For this review, take the finished solid that the model builds, in its own axes (mm). Face numbers are marked on the shaded views. Coordinates: 2 decimals unless noted, no trailing zeros. Loops run counter-clockwise (first coordinate to the right, second up) from the corner with the lowest first, then second, coordinate; pieces in that order, holes last.
```python
from build123d import *

# Parameters (mm, degrees)
SKETCH1_W           = 277
SKETCH1_H           = 3
BOSS_EXTRUDE1_DEPTH = 450
CUT_EXTRUDE1_REACH  = 520.295
SKETCH2_W           = 6
SKETCH2_H           = 250
CUT_EXTRUDE2_REACH  = 520.295
SKETCH3_R           = 1.55
SKETCH4_W           = 7
SKETCH4_H           = 75
SKETCH4_W_2         = 5
SKETCH4_H_2         = 35
BOSS_EXTRUDE2_DEPTH = 3


with BuildPart() as part:
    # Sketch1 → Boss-Extrude1 (new body)
    with BuildSketch(Plane.XY):
        with Locations((-118.640040599, -13.427850278)):
            Rectangle(SKETCH1_W, SKETCH1_H)
    extrude(amount=BOSS_EXTRUDE1_DEPTH)

    # Sketch2 → Cut-Extrude1 (cut, up to next)
    with BuildSketch(Plane(origin=(0, -11.927850278, 0), x_dir=(1, 0, 0), z_dir=(0, 1, 0)), mode=Mode.PRIVATE) as cut_extrude1_sk1:
        with Locations((-234.140040599, -225)):
            Rectangle(SKETCH2_W, SKETCH2_H)
    cut_extrude1_tool1 = extrude(cut_extrude1_sk1.sketch, amount=-CUT_EXTRUDE1_REACH, mode=Mode.PRIVATE) & part.part
    # Sketch2 → Cut-Extrude1 (cut, up to next)
    with BuildSketch(Plane(origin=(0, -11.927850278, 0), x_dir=(1, 0, 0), z_dir=(0, 1, 0)), mode=Mode.PRIVATE) as cut_extrude1_sk2:
        with Locations((-3.140040599, -225)):
            Rectangle(SKETCH2_W, SKETCH2_H)
    cut_extrude1_tool2 = extrude(cut_extrude1_sk2.sketch, amount=-CUT_EXTRUDE1_REACH, mode=Mode.PRIVATE) & part.part
    add(cut_extrude1_tool1.solids().sort_by_distance((-234.140041, -11.92785, 225))[0], mode=Mode.SUBTRACT)
    add(cut_extrude1_tool2.solids().sort_by_distance((-3.140041, -11.92785, 225))[0], mode=Mode.SUBTRACT)

    # Sketch3 → Cut-Extrude2 (cut, up to next)
    with BuildSketch(Plane(origin=(0, -11.927850278, 0), x_dir=(1, 0, 0), z_dir=(0, 1, 0)), mode=Mode.PRIVATE) as cut_extrude2_sk1:
        with Locations(Location((-102.460040599, -431.322984009, 0), (0, 0, 180))):
            Circle(SKETCH3_R)
    cut_extrude2_tool1 = extrude(cut_extrude2_sk1.sketch, amount=-CUT_EXTRUDE2_REACH, mode=Mode.PRIVATE) & part.part
    # Sketch3 → Cut-Extrude2 (cut, up to next)
    with BuildSketch(Plane(origin=(0, -11.927850278, 0), x_dir=(1, 0, 0), z_dir=(0, 1, 0)), mode=Mode.PRIVATE) as cut_extrude2_sk2:
        with Locations(Location((-75.460040599, -442.983238046, 0), (0, 0, 180))):
            Circle(SKETCH3_R)
    cut_extrude2_tool2 = extrude(cut_extrude2_sk2.sketch, amount=-CUT_EXTRUDE2_REACH, mode=Mode.PRIVATE) & part.part
    # Sketch3 → Cut-Extrude2 (cut, up to next)
    with BuildSketch(Plane(origin=(0, -11.927850278, 0), x_dir=(1, 0, 0), z_dir=(0, 1, 0)), mode=Mode.PRIVATE) as cut_extrude2_sk3:
        with Locations(Location((-92.910040599, -383.404829271, 0), (0, 0, 180))):
            Circle(SKETCH3_R)
    cut_extrude2_tool3 = extrude(cut_extrude2_sk3.sketch, amount=-CUT_EXTRUDE2_REACH, mode=Mode.PRIVATE) & part.part
    # Sketch3 → Cut-Extrude2 (cut, up to next)
    with BuildSketch(Plane(origin=(0, -11.927850278, 0), x_dir=(1, 0, 0), z_dir=(0, 1, 0)), mode=Mode.PRIVATE) as cut_extrude2_sk4:
        with Locations(Location((10.539959401, -350.404829271, 0), (0, 0, 180))):
            Circle(SKETCH3_R)
    cut_extrude2_tool4 = extrude(cut_extrude2_sk4.sketch, amount=-CUT_EXTRUDE2_REACH, mode=Mode.PRIVATE) & part.part
    # Sketch3 → Cut-Extrude2 (cut, up to next)
    with BuildSketch(Plane(origin=(0, -11.927850278, 0), x_dir=(1, 0, 0), z_dir=(0, 1, 0)), mode=Mode.PRIVATE) as cut_extrude2_sk5:
        with Locations(Location((-7.460040599, -444.433238046, 0), (0, 0, 180))):
            Circle(SKETCH3_R)
    cut_extrude2_tool5 = extrude(cut_extrude2_sk5.sketch, amount=-CUT_EXTRUDE2_REACH, mode=Mode.PRIVATE) & part.part
    # Sketch3 → Cut-Extrude2 (cut, up to next)
    with BuildSketch(Plane(origin=(0, -11.927850278, 0), x_dir=(1, 0, 0), z_dir=(0, 1, 0)), mode=Mode.PRIVATE) as cut_extrude2_sk6:
        with Locations(Location((-247.340040599, -350.40562763, 0), (0, 0, 180))):
            Circle(SKETCH3_R)
    cut_extrude2_tool6 = extrude(cut_extrude2_sk6.sketch, amount=-CUT_EXTRUDE2_REACH, mode=Mode.PRIVATE) & part.part
    # Sketch3 → Cut-Extrude2 (cut, up to next)
    with BuildSketch(Plane(origin=(0, -11.927850278, 0), x_dir=(1, 0, 0), z_dir=(0, 1, 0)), mode=Mode.PRIVATE) as cut_extrude2_sk7:
        with Locations(Location((-229.340040599, -444.434036405, 0), (0, 0, 180))):
            Circle(SKETCH3_R)
    cut_extrude2_tool7 = extrude(cut_extrude2_sk7.sketch, amount=-CUT_EXTRUDE2_REACH, mode=Mode.PRIVATE) & part.part
    # Sketch3 → Cut-Extrude2 (cut, up to next)
    with BuildSketch(Plane(origin=(0, -11.927850278, 0), x_dir=(1, 0, 0), z_dir=(0, 1, 0)), mode=Mode.PRIVATE) as cut_extrude2_sk8:
        with Locations(Location((-161.340040599, -442.984036405, 0), (0, 0, 180))):
            Circle(SKETCH3_R)
    cut_extrude2_tool8 = extrude(cut_extrude2_sk8.sketch, amount=-CUT_EXTRUDE2_REACH, mode=Mode.PRIVATE) & part.part
    # Sketch3 → Cut-Extrude2 (cut, up to next)
    with BuildSketch(Plane(origin=(0, -11.927850278, 0), x_dir=(1, 0, 0), z_dir=(0, 1, 0)), mode=Mode.PRIVATE) as cut_extrude2_sk9:
        with Locations(Location((-134.340040599, -431.323782367, 0), (0, 0, 180))):
            Circle(SKETCH3_R)
    cut_extrude2_tool9 = extrude(cut_extrude2_sk9.sketch, amount=-CUT_EXTRUDE2_REACH, mode=Mode.PRIVATE) & part.part
    # Sketch3 → Cut-Extrude2 (cut, up to next)
    with BuildSketch(Plane(origin=(0, -11.927850278, 0), x_dir=(1, 0, 0), z_dir=(0, 1, 0)), mode=Mode.PRIVATE) as cut_extrude2_sk10:
        with Locations(Location((-143.890040599, -383.40562763, 0), (0, 0, 180))):
            Circle(SKETCH3_R)
    cut_extrude2_tool10 = extrude(cut_extrude2_sk10.sketch, amount=-CUT_EXTRUDE2_REACH, mode=Mode.PRIVATE) & part.part
    add(cut_extrude2_tool1.solids().sort_by_distance((-102.460041, -11.92785, 431.322984))[0], mode=Mode.SUBTRACT)
    add(cut_extrude2_tool2.solids().sort_by_distance((-75.460041, -11.92785, 442.983238))[0], mode=Mode.SUBTRACT)
    add(cut_extrude2_tool3.solids().sort_by_distance((-92.910041, -11.92785, 383.404829))[0], mode=Mode.SUBTRACT)
    add(cut_extrude2_tool4.solids().sort_by_distance((10.539959, -11.92785, 350.404829))[0], mode=Mode.SUBTRACT)
    add(cut_extrude2_tool5.solids().sort_by_distance((-7.460041, -11.92785, 444.433238))[0], mode=Mode.SUBTRACT)
    add(cut_extrude2_tool6.solids().sort_by_distance((-247.340041, -11.92785, 350.405628))[0], mode=Mode.SUBTRACT)
    add(cut_extrude2_tool7.solids().sort_by_distance((-229.340041, -11.92785, 444.434036))[0], mode=Mode.SUBTRACT)
    add(cut_extrude2_tool8.solids().sort_by_distance((-161.340041, -11.92785, 442.984036))[0], mode=Mode.SUBTRACT)
    add(cut_extrude2_tool9.solids().sort_by_distance((-134.340041, -11.92785, 431.323782))[0], mode=Mode.SUBTRACT)
    add(cut_extrude2_tool10.solids().sort_by_distance((-143.890041, -11.92785, 383.405628))[0], mode=Mode.SUBTRACT)

    # Sketch4 → Boss-Extrude2 (add)
    with BuildSketch(Plane.XZ.offset(14.927850278)):
        with Locations((-253.640040599, 412.5)):
            Rectangle(SKETCH4_W, SKETCH4_H)
        with Locations((16.359959401, 412.5)):
            Rectangle(SKETCH4_W, SKETCH4_H)
        with Locations((-253.640040599, 37.5)):
            Rectangle(SKETCH4_W, SKETCH4_H)
        with Locations((16.359959401, 37.5)):
            Rectangle(SKETCH4_W, SKETCH4_H)
        with Locations((-118.640040599, 217.477852068)):
            Rectangle(SKETCH4_W_2, SKETCH4_H_2)
    extrude(amount=BOSS_EXTRUDE2_DEPTH)


solid = part.part
```
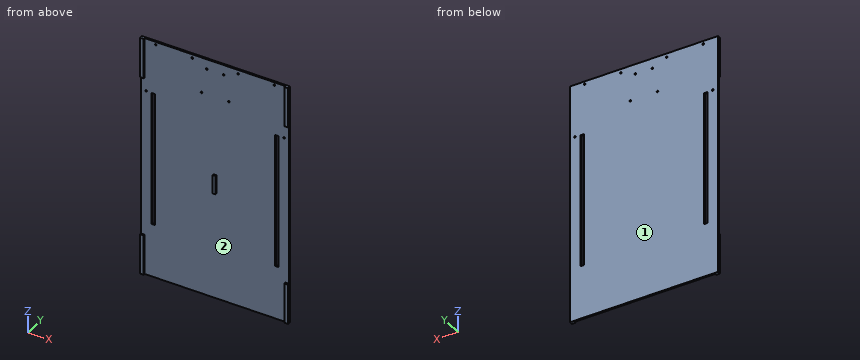
Q1. For pin 1 Ø3.5 at (x, y) = (-119.5, -17) entering from +Z; pin 2 Ø1.5 at (y, z) = (-17, 217.5) entering from -X; pin 3 Ø3.5 at (x, z) = (-143.89, 383.41) entering from -Y, all flat-tipped, find the tip position at first contact; note any pin that passes through.
Q2. Consider section B-B (z = 258). State the section outline as (x, y) points, then the cut area to 3 significant figures.
Q3. Consider section C-C (z = 403.5). State the section outline as (x, y) points, then the cut area to 3 significant figures.
Q4. Consider section A-A (y = -17). State the section outline as (x, z) points, then the cut area to 4 significant figures.
Q5. Wall thickness on probe 1 along X at (y, z) = (-12.25, 191.5); probe 2 along X at (y, z) = (-15, 24.5); probe 3 along Y at (x, z) = (-142.5, 246): over which ranges is each line inside the solid? List them lowest first.
Q6. The part is to be moulded in two halves that separate along X. For the marked faces 1 and 2, say which applies: +X half, -X half, draft (parallel to the pull), parting line (faces both ways), or undercut.
Q7. Consider section D-D (z = 208). State the section outline as (x, y) points, then the cut area to 3 significant figures.
Model answer:
1. pin 1: stops at z = 234.98
1. pin 2: stops at x = -121.14
1. pin 3: stops at y = -14.93
2. outline: (-257.14, -14.93) - (-237.14, -14.93) - (-237.14, -11.93) - (-257.14, -11.93) - close; (-231.14, -14.93) - (-6.14, -14.93) - (-6.14, -11.93) - (-231.14, -11.93) - close; (-0.14, -14.93) - (19.86, -14.93) - (19.86, -11.93) - (-0.14, -11.93) - close
2. area: 795 mm2
3. outline: (-257.14, -17.93) - (-250.14, -17.93) - (-250.14, -14.93) - (12.86, -14.93) - (12.86, -17.93) - (19.86, -17.93) - (19.86, -11.93) - (-257.14, -11.93) - close
3. area: 873 mm2
4. outline: (-257.14, 0) - (-250.14, 0) - (-250.14, 75) - (-257.14, 75) - close; (-257.14, 375) - (-250.14, 375) - (-250.14, 450) - (-257.14, 450) - close; (-121.14, 199.98) - (-116.14, 199.98) - (-116.14, 234.98) - (-121.14, 234.98) - close; (12.86, 0) - (19.86, 0) - (19.86, 75) - (12.86, 75) - close; (12.86, 375) - (19.86, 375) - (19.86, 450) - (12.86, 450) - close
4. area: 2,275 mm2
5. probe 1: x = -257.14 to -237.14, -231.14 to -6.14, -0.14 to 19.86
5. probe 2: x = -257.14 to -250.14, 12.86 to 19.86
5. probe 3: y = -14.93 to -11.93
6. face 1: draft
6. face 2: undercut
7. outline: (-257.14, -14.93) - (-237.14, -14.93) - (-237.14, -11.93) - (-257.14, -11.93) - close; (-231.14, -14.93) - (-121.14, -14.93) - (-121.14, -17.93) - (-116.14, -17.93) - (-116.14, -14.93) - (-6.14, -14.93) - (-6.14, -11.93) - (-231.14, -11.93) - close; (-0.14, -14.93) - (19.86, -14.93) - (19.86, -11.93) - (-0.14, -11.93) - close
7. area: 810 mm2
